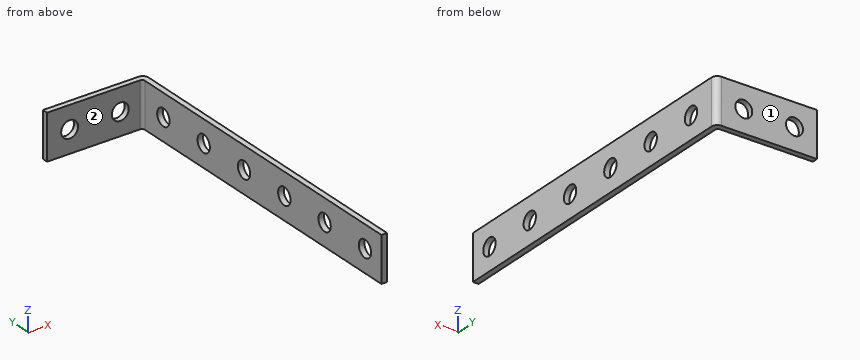
from build123d import *

# Parameters (mm, degrees)
F1_DEPTH = 8
F2_R     = 1.5
F3_DEPTH = 25
F4_R     = 1.5
F5_DEPTH = 25
F6_R     = 1
F7_R     = 0.5


with BuildPart() as f1:
    # F0 (on Top) → F1 (new body)
    with BuildSketch(Plane.XY):
        Polygon((-0.5, 29), (-0.5, -29), (0.5, -29), (0.5, 29), (0.5, 30), (-17.5, 30), (-17.5, 29), align=None)
    extrude(amount=F1_DEPTH)

    # F2 (on face) → F3 (cut)
    with BuildSketch(Plane(origin=(-0.5, 0, 0), x_dir=(0, -1, 0), z_dir=(-1, 0, 0))):
        with Locations((25, 4)):
            Circle(F2_R)
        with Locations((15.2, 4)):
            Circle(F2_R)
        with Locations((5.4, 4)):
            Circle(F2_R)
        with Locations((-4.4, 4)):
            Circle(F2_R)
        with Locations((-14.2, 4)):
            Circle(F2_R)
        with Locations((-24, 4)):
            Circle(F2_R)
    extrude(amount=-F3_DEPTH, mode=Mode.SUBTRACT)

    # F4 (on face) → F5 (cut)
    with BuildSketch(Plane.XZ.offset(-29)):
        with Locations((-4.5, 4)):
            Circle(F4_R)
        with Locations((-13.5, 4)):
            Circle(F4_R)
    extrude(amount=-F5_DEPTH, mode=Mode.SUBTRACT)

    # F6
    f6_edges = [f1.edges().sort_by_distance(p)[0] for p in [
        (0.5, 30, 4),
    ]]
    fillet(f6_edges, radius=F6_R)

    # F7
    f7_edges = [f1.edges().sort_by_distance(p)[0] for p in [
        (-0.5, 29, 4),
    ]]
    fillet(f7_edges, radius=F7_R)


solid = f1.part
Geometry: final body of the model. Coordinates: model frame, mm. Face numbers are marked on the shaded views. A direction names the side the tool comes from. Give positions to 0.01 mm unless a question says otherwise; leave off trailing zeros. Loops run counter-clockwise (first coordinate to the right, second up) from the corner with the lowest first, then second, coordinate; pieces in that order, holes last. Notation, with made-up numbers: M 86.5,-11.75 L 140.5,-11.75 A28 cw 140.5,23.25 Z; hole C -23.75,24.25 d3. An arc over 180 degrees is marked long. Put each result on its own line as item: value. Start each with the question number.
1) Cut plane C-C (z = 1.5). Output: boundary loops of the cut face in (x, y).
2) Contact query for flat-ended pins moving along their axis: pin 1 (2.5 mm diameter, centred on y = 24, z = 4, fed in from -X) (3 decimals); pin 2 (4 mm diameter, centred on x = -4.5, z = 4, fed in from +Y); pin 3 (4 mm diameter, centred on x = -13.5, z = 4, fed in from -Y); pin 4 (3 mm diameter, centred on y = 24, z = 6.5, fed in from -X). Output: stop coordinate, or through.
3) Cut plane A-A (x = -4.5). Output: boundary loops of the cut face in (y, z).
4) Cut plane B-B (y = 14.2). Output: boundary loops of the cut face in (x, z), then the cut area to 3 significant figures.
5) Cut plane D-D (y = 26). Output: boundary loops of the cut face in (x, z).
6) Access query for the marked faces 1 and 2. Directions: +Z, -Z, +X, -X, +Y, -Y. A direction counts if a zero-diameter tool reaches every point of the face in a straight line with its end or side. Return the directions, or none.
7) Ray query, line 1 along Z through (x, y) = (0, 4.4); line 2 along Y through (x, z) = (-3, 5); line 3 along X through (y, z) = (-6, 6.5). Return the intervals inside material, ascending.
Verdict:
1. outline: M -17.5,29 L -1,29 A0.5 cw -0.5,28.5 L -0.5,-29 L 0.5,-29 L 0.5,29 A1 ccw -0.5,30 L -17.5,30 Z
2. pin 1: through
2. pin 2: y = 30
2. pin 3: y = 29
2. pin 4: x = -0.5
3. outline: M 29,0 L 30,0 L 30,2.5 L 29,2.5 Z; M 29,5.5 L 30,5.5 L 30,8 L 29,8 Z
4. outline: M -0.5,0 L 0.5,0 L 0.5,2.5 L -0.5,2.5 Z; M -0.5,5.5 L 0.5,5.5 L 0.5,8 L -0.5,8 Z
4. area: 5.00 mm2
5. outline: M -0.5,0 L 0.5,0 L 0.5,8 L -0.5,8 Z
6. face 1: +Z, -Z, +X, -X, +Y
6. face 2: +Z, -Z, -X, -Y
7. line 1: 0 to 2.5, 5.5 to 8
7. line 2: 29 to 30
7. line 3: -0.5 to 0.5
